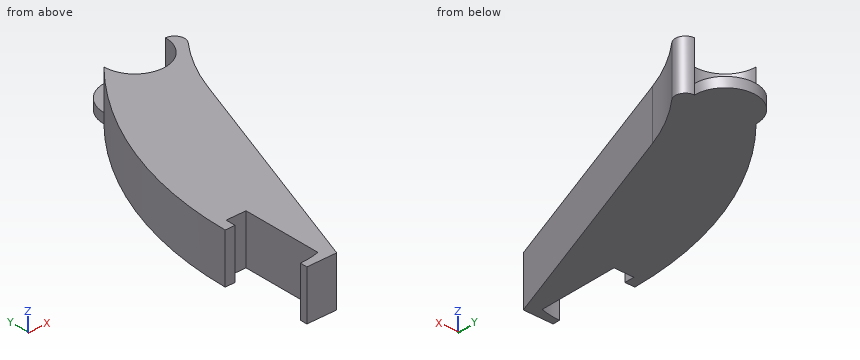
from build123d import *

# Parameters (mm, degrees)
F1_DEPTH = 25
F2_DEPTH = 5


with BuildPart() as f1:
    # F0 (on Top) → F1 (new body)
    with BuildSketch(Plane.XY):
        with BuildLine():
            Line((-10, 0), (0, 0))
            Line((0, 0), (0, -40))
            ThreePointArc((0, -40), (-4.9512, -41.048712), (-10, -41.400549))
            Line((-10, -41.400549), (-10, -45))
            Line((-10, -45), (5, -45))
            Line((5, -45), (48.925537, 75.68442))
            ThreePointArc((48.925537, 75.68442), (55.595415, 90.308655), (64.478844, 103.704185))
            ThreePointArc((64.478844, 103.704185), (65.043731, 109.03319), (60.5, 111.874299))
            ThreePointArc((60.5, 111.874299), (45, 96.374299), (29.5, 111.874299))
            ThreePointArc((29.5, 111.874299), (-3.498619, 57.529697), (-15, -5))
            Line((-15, -5), (-10, -5))
            Line((-10, -5), (-10, 0))
        make_face()
    extrude(amount=F1_DEPTH)

    # F0 (on Top) → F2 (join)
    with BuildSketch(Plane.XY):
        with BuildLine():
            Line((60.5, 111.874299), (29.5, 111.874299))
            ThreePointArc((29.5, 111.874299), (45, 96.374299), (60.5, 111.874299))
        make_face()
        with BuildLine():
            ThreePointArc((60.5, 111.874299), (45, 127.374299), (29.5, 111.874299))
            Line((29.5, 111.874299), (60.5, 111.874299))
        make_face()
    extrude(amount=F2_DEPTH)


solid = f1.part
The listing builds one solid part. Answer for the finished solid, in the listing's coordinates (mm). Give positions to 0.01 mm unless a question says otherwise; leave off trailing zeros. Order: outer loops, then holes, each group sorted by start corner. A loop starts at its lowest first (then second) coordinate and runs counter-clockwise, first axis right, second up. Notation, with made-up numbers: (15, 71.25) - (44, 71.25) arc R34 cw to (44, 105.25) - close; hole circle Ø10 at (88, 25.5). An arc over 180 degrees is marked (long way). Use one line per item in the form item = value.
1) Each of these flat-tipped pins is pushed along its axis until it touches: pin 1 (6 mm diameter, centred on y = 21, z = 4.5, fed in from -X); pin 2 (1.5 mm diameter, centred on y = 84, z = 9.5, fed in from +X); pin 3 (2 mm diameter, centred on y = 1, z = 19, fed in from +X). Where does it stop, or does it pass through?
Verdict:
pin_1 = -13.49
pin_2 = 52.73
pin_3 = 22.11
2) Find section D-D on x = 58.5. Determine the outline of the cut face in (y, z), and give its area (3 significant figures).
Verdict:
outline = (95.21, 0) - (119.49, 0) - (119.49, 5) - (104.26, 5) - (104.26, 25) - (95.21, 25) - close
area = 302 mm^2
3) Find section C-C on y = 40. Determine the outline of the cut face in (x, z).
Verdict:
outline = (-9.14, 0) - (35.94, 0) - (35.94, 25) - (-9.14, 25) - close
4) Find section B-B on x = 45. Determine the outline of the cut face in (y, z).
Verdict:
outline = (64.9, 0) - (127.37, 0) - (127.37, 5) - (96.37, 5) - (96.37, 25) - (64.9, 25) - close
5) Find section A-A on z = 7.75. Determine the outline of the cut face in (x, y).
Verdict:
outline = (-15, -5) - (-10, -5) - (-10, 0) - (0, 0) - (0, -40) arc R36.4 cw to (-10, -41.4) - (-10, -45) - (5, -45) - (48.93, 75.68) arc R102.05 cw to (64.48, 103.7) arc R5.05 ccw to (60.5, 111.87) arc R15.5 cw to (29.5, 111.87) arc R175.73 ccw to start
6) Consider probe 1 along X at (y, z) = (98, 7); probe 2 along X at (y, z) = (109.5, 15); probe 3 along X at (y, z) = (35, 19.5). Determine where each line is inside the solid, lowest interval first. Write a range as [from, to].
Verdict:
probe_1 = [18.35, 38.09], [51.91, 60.32]
probe_2 = [27.42, 29.68], [60.32, 64.79]
probe_3 = [-10.39, 34.12]
